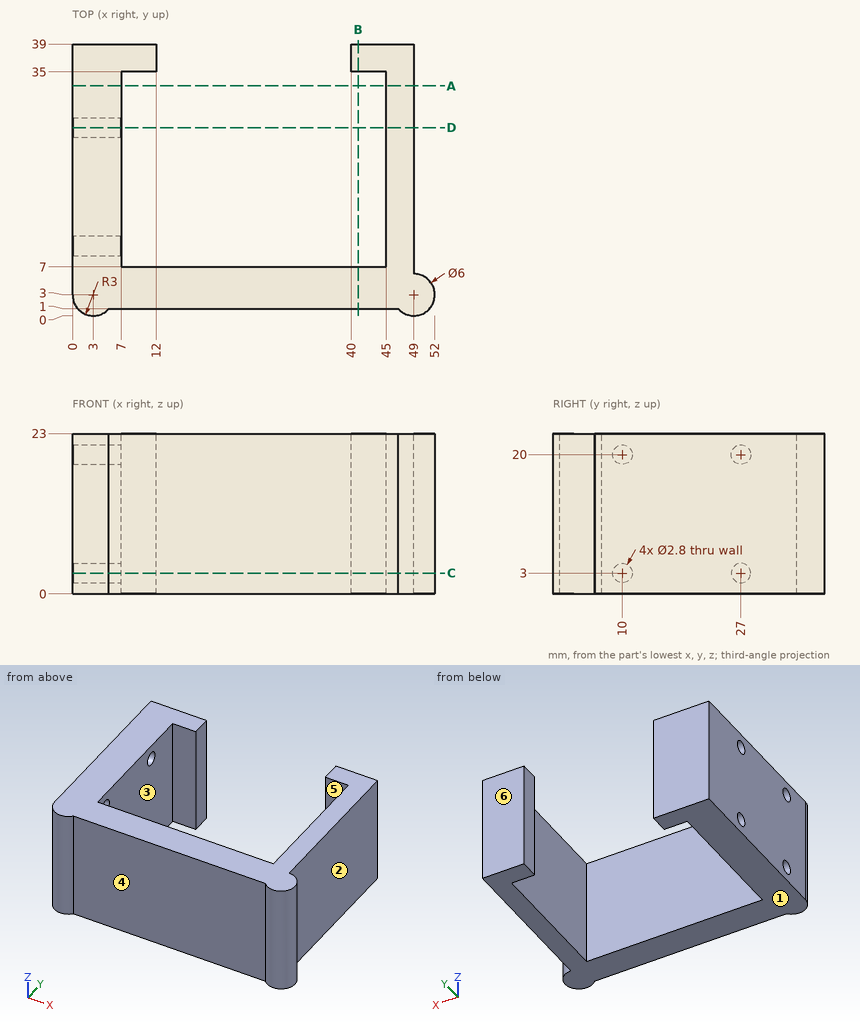
Can you work these out from the drawing? Everything is in mm from the part's minimum corner. A direction names the side the tool comes from. Give positions to 0.01 mm unless a question says otherwise; leave off trailing zeros. Write each loop counter-clockwise with the first axis right and the second up, starting at its lowest first coordinate (ties: lowest second). Pieces come first, ordered by that corner, then holes. Notation, with made-up numbers: (35, 76.25) -> (66, 76.25) arc R20 cw to (66, 114.25) -> close; hole circle Ø9 at (-27.5, 20). An arc over 180 degrees is marked (long way). Write each question's results on one line, items separated by ' | '. Start each with the question number.
Q1. Suppose I cut it at D-D, the plane y = 27. List the corners of the cut face in (x, z) for me.
Q2. Suppose I cut it at C-C, the plane z = 3. List the corners of the cut face in (x, y) for me.
Q3. Suppose I cut it at B-B, the plane x = 41. List the corners of the cut face in (y, z) for me, and give its area (3 significant figures).
Q4. I'm going to push flat-ended pins straight in: pin 1 Ø3 at (x, z) = (36, 4) entering from +Y; pin 2 Ø5 at (x, z) = (44.5, 8.5) entering from -Y; pin 3 Ø5.5 at (x, z) = (9.5, 14.5) entering from -Y. Where does each tip first touch, or does it pass through?
Q5. I need wall thicknesses on probe 1 along X at (y, z) = (33, 2); probe 2 along Z at (x, y) = (3.75, 27); probe 3 along Y at (x, z) = (3.5, 20). Which ranges of each line are inside material? Lowest first, please.
Q6. Which directions (+Z, -Z, +X, -X, +Y, -Y) give clear straight access to the entire face, cutting with the end or side of a thin tool? Please do the marked faces 4, 5 and 6.
Q7. We'd pull the mould along X, two halves only. Please class the marked faces 1, 2 and 3: +X half, -X half, draft (parallel to the pull), parting line (faces both ways), or undercut.
Q8. Suppose I cut it at A-A, the plane y = 33. List the corners of the cut face in (x, z) for me.
Outcome:
1) outline: (0, 0) -> (7, 0) -> (7, 1.6) -> (0, 1.6) -> close; (0, 4.4) -> (7, 4.4) -> (7, 18.6) -> (0, 18.6) -> close; (0, 21.4) -> (7, 21.4) -> (7, 23) -> (0, 23) -> close; (45, 0) -> (49, 0) -> (49, 23) -> (45, 23) -> close
2) outline: (0, 3) arc R3 ccw to (5.24, 1) -> (46.76, 1) arc R3 ccw (long way) to (49, 6) -> (49, 39) -> (40, 39) -> (40, 35) -> (45, 35) -> (45, 7) -> (7, 7) -> (7, 8.6) -> (0, 8.6) -> close; (0, 11.4) -> (7, 11.4) -> (7, 25.6) -> (0, 25.6) -> close; (0, 28.4) -> (7, 28.4) -> (7, 35) -> (12, 35) -> (12, 39) -> (0, 39) -> close
3) outline: (1, 0) -> (7, 0) -> (7, 23) -> (1, 23) -> close; (35, 0) -> (39, 0) -> (39, 23) -> (35, 23) -> close | area: 230 mm2
4) pin 1: y = 7 | pin 2: y = 0.76 | pin 3: y = 1
5) probe 1: 0 to 7, 45 to 49 | probe 2: 0 to 1.6, 4.4 to 18.6, 21.4 to 23 | probe 3: 0.04 to 8.6, 11.4 to 25.6, 28.4 to 39
6) face 4: +Z, -Z, -Y | face 5: +Z, -Z | face 6: +Z, -Z, +X, -X, +Y
7) face 1: draft | face 2: +X half | face 3: undercut
8) outline: (0, 0) -> (7, 0) -> (7, 23) -> (0, 23) -> close; (45, 0) -> (49, 0) -> (49, 23) -> (45, 23) -> close
